```python
from build123d import *

# Parameters (mm, degrees)
SKETCH1_W           = 30.48
SKETCH1_H           = 47.625
BOSS_EXTRUDE1_DEPTH = 50.8
CUT_EXTRUDE1_DEPTH  = 50.8
FILLET1_R           = 2.54
FILLET2_R           = 2.54
BOSS_EXTRUDE2_DEPTH = 25.4
SKETCH4_W           = 10.16
SKETCH4_H           = 20.32
BOSS_EXTRUDE3_DEPTH = 25.4


with BuildPart() as part:
    # Sketch1 → Boss-Extrude1 (new body)
    with BuildSketch(Plane(origin=(0, 0, 0), x_dir=(1, 0, 0), z_dir=(0, 1, 0))):
        Rectangle(SKETCH1_W, SKETCH1_H)
    extrude(amount=BOSS_EXTRUDE1_DEPTH)

    # Sketch2 → Cut-Extrude1 (cut)
    with BuildSketch(Plane(origin=(0, 50.8, 0), x_dir=(1, 0, 0), z_dir=(0, 1, 0))):
        Polygon((3.302, -5.159375), (-3.302, 5.159375), (-3.302, 0), (-3.302, -11.1125), (3.302, -11.1125), align=None)
        Polygon((-3.302, 11.1125), (-3.302, 5.159375), (3.302, -5.159375), (3.302, 0), (3.302, 11.1125), (0, 11.1125), align=None)
    extrude(amount=-CUT_EXTRUDE1_DEPTH, mode=Mode.SUBTRACT)

    # Fillet1
    fillet1_edges = [part.edges().sort_by_distance(p)[0] for p in [
        (-3.302, 25.4, 11.1125),
        (-3.302, 25.4, -11.1125),
        (3.302, 25.4, -11.1125),
        (3.302, 25.4, 11.1125),
    ]]
    fillet(fillet1_edges, radius=FILLET1_R)

    # Fillet2
    fillet2_edges = [part.edges().sort_by_distance(p)[0] for p in [
        (15.24, 25.4, 23.8125),
        (-15.24, 25.4, 23.8125),
        (-15.24, 25.4, -23.8125),
        (15.24, 25.4, -23.8125),
    ]]
    fillet(fillet2_edges, radius=FILLET2_R)

    # Sketch3 → Boss-Extrude2 (add)
    with BuildSketch(Plane(origin=(0, 0, -23.8125), x_dir=(-1, 0, 0), z_dir=(0, 0, -1))):
        Polygon((-5.080578249, 35.561156499), (-5.080578249, 15.238843501), (5.080578249, 35.561156499), align=None)
        Polygon((5.080578249, 35.561156499), (-5.080578249, 15.238843501), (5.080578249, 15.238843501), align=None)
    extrude(amount=BOSS_EXTRUDE2_DEPTH)

    # Sketch4 → Boss-Extrude3 (add)
    with BuildSketch(Plane.XY.offset(23.8125)):
        with Locations((0, 25.4)):
            Rectangle(SKETCH4_W, SKETCH4_H)
    extrude(amount=BOSS_EXTRUDE3_DEPTH)


solid = part.part
```
Could you check a few things on this model? Use its own coordinates, in mm. A direction names the side the tool comes from. Coordinates: 2 decimals unless noted, no trailing zeros. Loops run counter-clockwise (first coordinate to the right, second up) from the corner with the lowest first, then second, coordinate; pieces in that order, holes last. Notation, with made-up numbers: M 9.5,4 L 41.5,4 A16 ccw 41.5,33 Z; hole C 10.5,8 d2. An arc over 180 degrees is marked long. Put each result on its own line as item: value. Start each with the question number.
(1) Suppose I cut it at B-B on y = 38. Please give me the cut outline in (x, z).
(2) I need wall thicknesses on line 1 (Z direction, x = 9.5, y = 6.5); line 2 (X direction, y = 46.5, z = 5); line 3 (Z direction, x = -1.5, y = 21). Which ranges of each line are inside material? Lowest first, please. Write a range as from..to.
(3) Suppose I cut it at A-A on z = -5. Please give me the cut outline in (x, y), then the cut area to 3 significant figures.
(4) Will these pins go through, and if not, where does the flat tip stop? P1, Ø10, axis at x = 8, z = 38, coming from the +Y side; P2, Ø1.5, axis at x = 6.5, y = 44, coming from the +Z side; P3, Ø16.5, axis at y = 23.5, z = 39.5, coming from the +X side.
(5) Suppose I cut it at C-C on x = -6.5. Please give me the cut outline in (y, z).
(6) Suppose I cut it at D-D on z = 37.5. Please give me the cut outline in (x, y), then the cut area to 3 significant figures.
(7) For faces 5 (the face through (5.08, 25, 36)), 6 (the face through (0, 15.239, -36)), 7 (the face through (-5.081, 25, -36)), which set-ups out of +Z, -Z, +X, -X, +Y, -Y let a thin tool reach every point of the face, with its end or its side?
(8) Thinking about a two-plate mould opening in Z: for faces 1 (the face through (-14.516, 25.756, -23.049)), 2 (the face through (0, 35.56, 36)), 3 (the face through (-3.302, 26, 0)), 4 (the face through (3.302, 26, 0)), which applies, pulls with the +Z half, pulls with the -Z half, needs draft (parallel to the pull), parting line crosses it, or undercut?
Solutions:
1. outline: M -15.24,-21.27 A2.54 ccw -12.7,-23.81 L 12.7,-23.81 A2.54 ccw 15.24,-21.27 L 15.24,21.27 A2.54 ccw 12.7,23.81 L -12.7,23.81 A2.54 ccw -15.24,21.27 Z; hole M -3.3,-8.57 A2.54 ccw -0.76,-11.11 L 0.76,-11.11 A2.54 ccw 3.3,-8.57 L 3.3,8.57 A2.54 ccw 0.76,11.11 L -0.76,11.11 A2.54 ccw -3.3,8.57 Z
2. line 1: z = -23.81..23.81
2. line 2: x = -15.24..-3.3, 3.3..15.24
2. line 3: z = -49.21..-11, 11..49.21
3. outline: M -15.24,0 L -3.3,0 L -3.3,50.8 L -15.24,50.8 Z; M 3.3,0 L 15.24,0 L 15.24,50.8 L 3.3,50.8 Z
3. area: 1,210 mm2
4. P1: stops at y = 35.56
4. P2: stops at z = 23.81
4. P3: stops at x = 5.08
5. outline: M 0,-23.81 L 50.8,-23.81 L 50.8,23.81 L 0,23.81 Z
6. outline: M -5.08,15.24 L 5.08,15.24 L 5.08,35.56 L -5.08,35.56 Z
6. area: 206 mm2
7. face 5: +Z, +X, +Y, -Y
7. face 6: -Z, +X, -X, -Y
7. face 7: -Z, -X, +Y, -Y
8. face 1: pulls with the -Z half
8. face 2: needs draft
8. face 3: undercut
8. face 4: undercut
